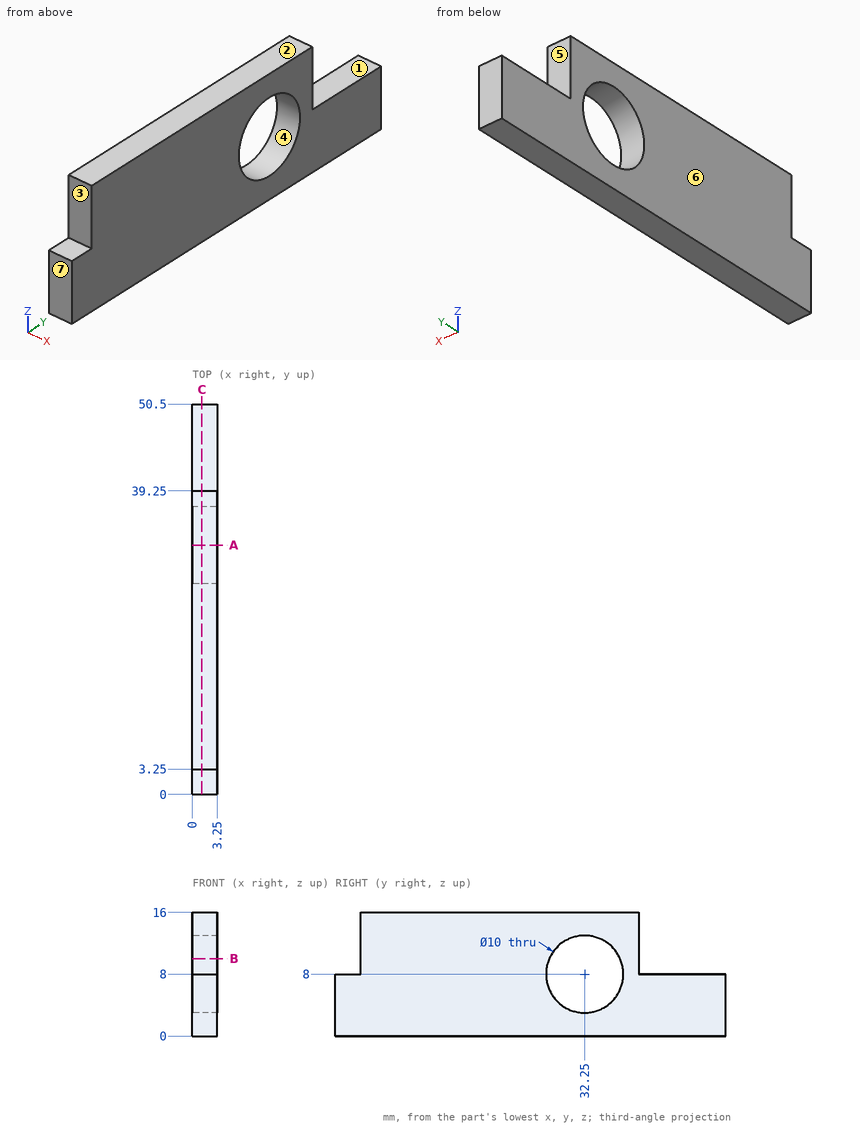
For this review, use the dimensioned drawing (mm, ordinates from the lowest corner) and the shaded views. A direction names the side the tool comes from. Coordinates: 2 decimals unless noted, no trailing zeros. Write each loop counter-clockwise with the first axis right and the second up, starting at its lowest first coordinate (ties: lowest second). Pieces come first, ordered by that corner, then holes. Notation, with made-up numbers: (-12, 9) - (17, 9) arc R15 cw to (17, 22) - close; hole circle Ø4 at (49, 67). An arc over 180 degrees is marked (long way). Answer as a JSON object with one key per item and string values. Group by question number.
1. Add section B-B (z = 10). Give the boundary of the cut face in (x, y), plus the area to 3 significant figures.
2. Add section A-A (y = 32.25). Give the boundary of the cut face in (x, z), plus the area to 3 significant figures.
3. Clearance check with flat-ended pins moving along their axes: pin 1 Ø1 at (x, z) = (1, 11) entering from +Y; pin 2 Ø8 at (y, z) = (32.25, 8) entering from +X. State where each tip first meets the part, or that it passes through.
4. Machinability: for the marked faces 1, 2 and 3, which of the approach directions +Z, -Z, +X, -X, +Y, -Y give a long, thin tool a straight path to every point of the face, cutting with its end or side? Answer none if there is none.
5. Mouldability with a two-part tool opening along Y and no side actions: class the marked faces 4, 5, 6 and 7 as pulls with the +Y half, pulls with the -Y half, needs draft (parallel to the pull), parting line crosses it, or undercut.
6. Add section C-C (x = 1.25). Give the boundary of the cut face in (y, z).
7. To check wall thickness, follow probe 1 along Z at (x, y) = (2.35, 32.25); probe 2 along Z at (x, y) = (2.5, 40.5); probe 3 along Y at (x, z) = (0.9, 5.5). State the ranges of each line that lie inside material, in increasing order.
Findings:
{
 "1": {"outline": "(0, 3.25) - (3.25, 3.25) - (3.25, 27.67) - (0, 27.67) - close; (0, 36.83) - (3.25, 36.83) - (3.25, 39.25) - (0, 39.25) - close", "area": "87.2 mm²"},
 "2": {"outline": "(0, 0) - (3.25, 0) - (3.25, 3) - (0, 3) - close; (0, 13) - (3.25, 13) - (3.25, 16) - (0, 16) - close", "area": "19.5 mm²"},
 "3": {"pin 1": "y = 39.25", "pin 2": "through"},
 "4": {"face 1": "+Z, +X, -X, +Y", "face 2": "+Z, +X, -X, +Y, -Y", "face 3": "+Z, +X, -X, -Y"},
 "5": {"face 4": "undercut", "face 5": "pulls with the +Y half", "face 6": "needs draft", "face 7": "pulls with the -Y half"},
 "6": {"outline": "(0, 0) - (50.5, 0) - (50.5, 8) - (39.25, 8) - (39.25, 16) - (3.25, 16) - (3.25, 8) - (0, 8) - close; hole circle Ø10 at (32.25, 8)"},
 "7": {"probe 1": "0 to 3, 13 to 16", "probe 2": "0 to 8", "probe 3": "0 to 27.92, 36.58 to 50.5"}
}
